from build123d import *

# Parameters (mm, degrees)
BOSS_EXTRUDE1_DEPTH = 9
SKETCH6_15_R        = 9
CUT_EXTRUDE1_DEPTH  = 188.397972241
SKETCH6_17_R        = 11
CUT_EXTRUDE2_DEPTH  = 7
CUT_EXTRUDE3_START  = 9
CUT_EXTRUDE3_DEPTH  = 6


with BuildPart() as part:
    # Sketch6 → Boss-Extrude1 (new body)
    with BuildSketch(Plane.XY):
        with BuildLine():
            Line((11.124297731, -11.5), (163.700491182, -20.95975374))
            ThreePointArc((163.700491182, -20.95975374), (186, 0), (163.700491182, 20.95975374))
            Line((163.700491182, 20.95975374), (11.124297731, 11.5))
            ThreePointArc((11.124297731, 11.5), (-16, 0), (11.124297731, -11.5))
        make_face()
    extrude(amount=BOSS_EXTRUDE1_DEPTH)

    # Sketch6<15> → Cut-Extrude1 (cut, through all)
    with BuildSketch(Plane.XY):
        with Locations((165, 0)):
            Circle(SKETCH6_15_R)
        Circle(SKETCH6_15_R)
    extrude(amount=CUT_EXTRUDE1_DEPTH, mode=Mode.SUBTRACT)

    # Sketch6<17> → Cut-Extrude2 (cut)
    with BuildSketch(Plane.XY):
        with Locations((165, 0)):
            Circle(SKETCH6_17_R)
        Circle(SKETCH6_17_R)
    extrude(amount=CUT_EXTRUDE2_DEPTH, mode=Mode.SUBTRACT)

    # Sketch6<18> → Cut-Extrude3 (cut)
    with BuildSketch(Plane.XY.offset(CUT_EXTRUDE3_START)):
        with BuildLine():
            Line((28.572170682, 7.572170682), (125.447559308, 13.552440692))
            ThreePointArc((125.447559308, 13.552440692), (139, 0), (125.447559308, -13.552440692))
            Line((125.447559308, -13.552440692), (28.572170682, -7.572170682))
            ThreePointArc((28.572170682, -7.572170682), (21, 0), (28.572170682, 7.572170682))
        make_face()
    extrude(amount=-CUT_EXTRUDE3_DEPTH, mode=Mode.SUBTRACT)


solid = part.part
Could you check a few things on this model? Use its own coordinates, in mm. A direction names the side the tool comes from. Give positions to 0.01 mm unless a question says otherwise; leave off trailing zeros. Order: outer loops, then holes, each group sorted by start corner. A loop starts at its lowest first (then second) coordinate and runs counter-clockwise, first axis right, second up.
Item 1: If we mould it in two halves opening along X, with no side actions, what happens to faces 4 (the face through (106, 0, 0)), 5 (the face through (139, 0, 6))? For each: pulls with the +X half, pulls with the -X half, needs draft (parallel to the pull), parting line crosses it, or undercut.
Item 2: If we section it at C-C, the plane x = 72: Write out the boundary of the cut face in (y, z), plus the area to 3 significant figures.
Item 3: If we section it at B-B, the plane y = 0: Write out the boundary of the cut face in (x, z), plus the area to 3 significant figures.
Item 4: I'm going to push flat-ended pins straight in: pin 1 (6 mm diameter, centred on x = 23, y = 6.5, fed in from -Z); pin 2 (1 mm diameter, centred on y = 0, z = 6.5, fed in from +X); pin 3 (2 mm diameter, centred on y = 16, z = 4, fed in from +X); pin 4 (2 mm diameter, centred on x = 15, z = 5, fed in from -Y). Where does each tip first touch, or does it pass through?
Item 5: If we section it at A-A, the plane x = 0: Write out the boundary of the cut face in (y, z), plus the area to 3 significant figures.
Item 6: If we section it at D-D, the plane x = 131: Write out the boundary of the cut face in (y, z).
Item 7: I need wall thicknesses on line 1 (X direction, y = 0, z = 8.45); line 2 (Y direction, x = 0, z = 8.6); line 3 (Y direction, x = 0, z = 4.5). Which ranges of each line are inside material? Lowest first, please.
Item 8: For faces 1 (the face through (77.688, -10.604, 6.042)), 2 (the face through (2, -9, 7)), 3 (the face through (88.48, 16.296, 4.437)), which set-ups out of +Z, -Z, +X, -X, +Y, -Y let a thin tool reach every point of the face, with its end or its side?
Values:
1. face 4: needs draft
1. face 5: undercut
2. outline: (-15.27, 0) - (15.27, 0) - (15.27, 9) - (10.25, 9) - (10.25, 3) - (-10.25, 3) - (-10.25, 9) - (-15.27, 9) - close
2. area: 152 mm2
3. outline: (-16, 0) - (-11, 0) - (-11, 7) - (-9, 7) - (-9, 9) - (-16, 9) - close; (9, 7) - (11, 7) - (11, 0) - (154, 0) - (154, 7) - (156, 7) - (156, 9) - (139, 9) - (139, 3) - (21, 3) - (21, 9) - (9, 9) - close; (174, 7) - (176, 7) - (176, 0) - (186, 0) - (186, 9) - (174, 9) - close
3. area: 730 mm2
4. pin 1: stops at z = 0
4. pin 2: stops at x = 186
4. pin 3: stops at x = 179.7
4. pin 4: stops at y = -11.8
5. outline: (-16, 0) - (-11, 0) - (-11, 7) - (-9, 7) - (-9, 9) - (-16, 9) - close; (9, 7) - (11, 7) - (11, 0) - (16, 0) - (16, 9) - (9, 9) - close
5. area: 98.0 mm2
6. outline: (-18.93, 0) - (18.93, 0) - (18.93, 9) - (12.36, 9) - (12.36, 3) - (-12.36, 3) - (-12.36, 9) - (-18.93, 9) - close
7. line 1: x = -16 to -9, 9 to 21, 139 to 156, 174 to 186
7. line 2: y = -16 to -9, 9 to 16
7. line 3: y = -16 to -11, 11 to 16
8. face 1: +Z
8. face 2: -Z
8. face 3: +Z, -Z, +Y
